Can you work these out from the model? Positions are in its coordinate system, mm. Coordinates: 2 decimals unless noted, no trailing zeros. Order: outer loops, then holes, each group sorted by start corner. A loop starts at its lowest first (then second) coordinate and runs counter-clockwise, first axis right, second up. Notation, with made-up numbers: (31.25, 62) -> (37.25, 62) arc R14 ccw to (37.25, 68) -> close; hole circle Ø3 at (82, 71.5). An arc over 180 degrees is marked (long way). Use a Markdown table: item, result. Add a question column.
1. Suppose I cut it at D-D, the plane y = 116.5. List the corners of the cut face in (x, z) for me.
2. For pin 1 Ø0.6 at (y, z) = (172, 1) entering from -X, with a flat end and sliding along its axis, tell me the tip position at first contact or that it passes through.
3. If I drill on line 1 along Y through (x, z) = (0, 0.85); line 2 along Y through (x, z) = (-2.5, 0.8); line 3 along X through (y, z) = (83, 0.4), over which ranges is the centre line in solid material (lowest first)? Write a range as from..to.
4. Suppose I cut it at B-B, the plane x = 0. List the corners of the cut face in (y, z) for me.
5. We'd pull the mould along Y, two halves only. Please class faces 1 (the cylindrical face through (-0.175, 42.835, 0.791)), 2 (the flat face through (0, 121, 0)), 3 (the flat face through (-12.175, 103.952, 0.769)): pulls with the +Y half, pulls with the -Y half, needs draft (parallel to the pull), parting line crosses it, or undercut.
6. Suppose I cut it at A-A, the plane z = 0.85. List the corners of the cut face in (x, y) for me, then the cut area to 3 significant figures.
7. Suppose I cut it at C-C, the plane y = 41.5. List the corners of the cut face in (x, z) for me.
```python
from build123d import *

# Parameters (mm, degrees)
EXTRUDE1_DEPTH     = 1.56
SKETCH2_R          = 1.3462
CUT_EXTRUDE2_DEPTH = 2.56
EXTRUDE2_DEPTH     = 1.56
FILLET1_R          = 0.5
SKETCH5_R          = 0.396875
EXTRUDE3_DEPTH     = 2.56


with BuildPart() as part:
    # Sketch1 → Extrude1 (new body)
    with BuildSketch(Plane.XY):
        Polygon((-7.655500537, 35), (7.655500537, 35), (16.56941148, 171), (-16.56941148, 171), align=None)
    extrude(amount=EXTRUDE1_DEPTH)

    # Sketch2 → Cut-Extrude2 (cut, through all)
    with BuildSketch(Plane(origin=(2.513247729, -24.95744912, 1.56), x_dir=(1, 0, 0), z_dir=(0, 0, 1))):
        with Locations((-2.513247729, 66.45744912)):
            Circle(SKETCH2_R)
    extrude(amount=-CUT_EXTRUDE2_DEPTH, mode=Mode.SUBTRACT)

    # Sketch4 → Extrude2 (add)
    with BuildSketch(Plane(origin=(0, 0, 0), x_dir=(-1, 0, 0), z_dir=(0, 0, -1))):
        with BuildLine():
            Line((-16.56941148, 171), (-16.628059301, 171.894792828))
            ThreePointArc((-16.628059301, 171.894792828), (-14.720969619, 173.99894204), (-12.68034522, 172.024027605))
            Line((-12.68034522, 172.024027605), (-12.68034522, 171))
            Line((-12.68034522, 171), (-16.56941148, 171))
        make_face()
    extrude(amount=-EXTRUDE2_DEPTH)

    # Fillet1
    fillet1_edges = [part.edges().sort_by_distance(p)[0] for p in [
        (12.68034522, 171, 0.78),
    ]]
    fillet(fillet1_edges, radius=FILLET1_R)

    # Sketch5 → Extrude3 (cut, through all)
    with BuildSketch(Plane.XY.offset(1.56)):
        with Locations((14.656317615, 172.024027605)):
            Circle(SKETCH5_R)
    extrude(amount=-EXTRUDE3_DEPTH, mode=Mode.SUBTRACT)


solid = part.part
```
Worked out:
| question | item | result |
|---|---|---|
| 1 | outline | (-13, 0) -> (13, 0) -> (13, 1.56) -> (-13, 1.56) -> close |
| 2 | pin 1 | stops at x = 12.68 |
| 3 | line 1 | y = 35..40.15, 42.85..171 |
| 3 | line 2 | y = 35..171 |
| 3 | line 3 | x = -10.8..10.8 |
| 4 | outline | (35, 0) -> (40.15, 0) -> (40.15, 1.56) -> (35, 1.56) -> close; (42.85, 0) -> (171, 0) -> (171, 1.56) -> (42.85, 1.56) -> close |
| 5 | face 1 | undercut |
| 5 | face 2 | needs draft |
| 5 | face 3 | pulls with the -Y half |
| 6 | outline | (-16.57, 171) -> (-7.66, 35) -> (7.66, 35) -> (16.63, 171.89) arc R1.98 ccw (long way) to (12.68, 172.02) -> (12.68, 171.5) arc R0.5 cw to (12.18, 171) -> close; hole circle Ø2.69 at (0, 41.5); hole circle Ø0.79 at (14.66, 172.02) |
| 6 | area | 3,300 mm² |
| 7 | outline | (-8.08, 0) -> (-1.35, 0) -> (-1.35, 1.56) -> (-8.08, 1.56) -> close; (1.35, 0) -> (8.08, 0) -> (8.08, 1.56) -> (1.35, 1.56) -> close |
